```python
from build123d import *

# Parameters (mm, degrees)
F1_DEPTH      = 5
F2_ANGLE      = 30
F0_R          = 15
F4_DEPTH      = 25
F4_DEPTH_BACK = 25
F5_COUNT      = 6
F6_DEPTH      = 8.3061645655
F6_DEPTH_BACK = 8.3061645655


with BuildPart() as f1:
    # F0 (on Top) → F1 (new body, symmetric)
    with BuildSketch(Plane.XY):
        with BuildLine():
            Line((28.9777747887, -7.7645713531), (96.5925826289, -25.8819045103))
            ThreePointArc((96.5925826289, -25.8819045103), (100, 0), (96.5925826289, 25.8819045103))
            Line((96.5925826289, 25.8819045103), (28.9777747887, 7.7645713531))
            ThreePointArc((28.9777747887, 7.7645713531), (29.7433458412, 3.9157857666), (30, 0))
            ThreePointArc((30, 0), (29.7433458412, -3.9157857666), (28.9777747887, -7.7645713531))
        make_face()
        with BuildLine():
            Line((23.4384574105, -6.280315735), (28.9777747887, -7.7645713531))
            ThreePointArc((28.9777747887, -7.7645713531), (29.7433458412, -3.9157857666), (30, 0))
            ThreePointArc((30, 0), (29.7433458412, 3.9157857666), (28.9777747887, 7.7645713531))
            Line((28.9777747887, 7.7645713531), (23.4384574105, 6.280315735))
            ThreePointArc((23.4384574105, 6.280315735), (24.2652766627, 0), (23.4384574105, -6.280315735))
        make_face()
    extrude(amount=F1_DEPTH, both=True)


with BuildPart() as f1_1:
    # F2: moved
    add(f1.part.rotate(Axis((53.4821525216, 0, 0), (1, 0, 0)), F2_ANGLE))

    # F0 (on Top) → F4 (cut, two sides)
    with BuildSketch(Plane.XY) as f4_sk:
        with BuildLine():
            ThreePointArc((28.9777747887, 7.7645713531), (-30, 0), (28.9777747887, -7.7645713531))
            Line((28.9777747887, -7.7645713531), (23.4384574105, -6.280315735))
            ThreePointArc((23.4384574105, -6.280315735), (24.2652766627, 0), (23.4384574105, 6.280315735))
            Line((23.4384574105, 6.280315735), (28.9777747887, 7.7645713531))
        make_face()
        Circle(F0_R, mode=Mode.SUBTRACT)
        with BuildLine():
            Line((23.4384574105, -6.280315735), (28.9777747887, -7.7645713531))
            ThreePointArc((28.9777747887, -7.7645713531), (29.7433458412, -3.9157857666), (30, 0))
            ThreePointArc((30, 0), (29.7433458412, 3.9157857666), (28.9777747887, 7.7645713531))
            Line((28.9777747887, 7.7645713531), (23.4384574105, 6.280315735))
            ThreePointArc((23.4384574105, 6.280315735), (24.2652766627, 0), (23.4384574105, -6.280315735))
        make_face()
    extrude(amount=-F4_DEPTH, mode=Mode.SUBTRACT)
    extrude(f4_sk.sketch, amount=F4_DEPTH_BACK, mode=Mode.SUBTRACT)


with BuildPart() as f5_1:
    # F5: instance of F1
    add(f1_1.part.rotate(Axis((0, 0, 24.5690848678), (0, 0, 1)), 1 * 360 / F5_COUNT))


with BuildPart() as f5_2:
    # F5: instance of F1
    add(f1_1.part.rotate(Axis((0, 0, 24.5690848678), (0, 0, 1)), 2 * 360 / F5_COUNT))


with BuildPart() as f5_3:
    # F5: instance of F1
    add(f1_1.part.rotate(Axis((0, 0, 24.5690848678), (0, 0, 1)), 3 * 360 / F5_COUNT))


with BuildPart() as f5_4:
    # F5: instance of F1
    add(f1_1.part.rotate(Axis((0, 0, 24.5690848678), (0, 0, 1)), 4 * 360 / F5_COUNT))


with BuildPart() as f5_5:
    # F5: instance of F1
    add(f1_1.part.rotate(Axis((0, 0, 24.5690848678), (0, 0, 1)), 5 * 360 / F5_COUNT))


with BuildPart() as f1_2:
    add(f1_1.part)

    add(f5_1.part)  # F6 merges F5_1

    add(f5_2.part)  # F6 merges F5_2

    add(f5_3.part)  # F6 merges F5_3

    add(f5_4.part)  # F6 merges F5_4

    add(f5_5.part)  # F6 merges F5_5
    # F0 (on Top) → F6 (join, two sides)
    with BuildSketch(Plane.XY) as f6_sk:
        with BuildLine():
            ThreePointArc((28.9777747887, 7.7645713531), (-30, 0), (28.9777747887, -7.7645713531))
            Line((28.9777747887, -7.7645713531), (23.4384574105, -6.280315735))
            ThreePointArc((23.4384574105, -6.280315735), (24.2652766627, 0), (23.4384574105, 6.280315735))
            Line((23.4384574105, 6.280315735), (28.9777747887, 7.7645713531))
        make_face()
        Circle(F0_R, mode=Mode.SUBTRACT)
        with BuildLine():
            Line((23.4384574105, -6.280315735), (28.9777747887, -7.7645713531))
            ThreePointArc((28.9777747887, -7.7645713531), (29.7433458412, -3.9157857666), (30, 0))
            ThreePointArc((30, 0), (29.7433458412, 3.9157857666), (28.9777747887, 7.7645713531))
            Line((28.9777747887, 7.7645713531), (23.4384574105, 6.280315735))
            ThreePointArc((23.4384574105, 6.280315735), (24.2652766627, 0), (23.4384574105, -6.280315735))
        make_face()
    extrude(amount=F6_DEPTH)
    extrude(f6_sk.sketch, amount=-F6_DEPTH_BACK)


solid = f1_2.part
```
Could you check a few things on this model? Use its own coordinates, in mm. A direction names the side the tool comes from. Coordinates: 2 decimals unless noted, no trailing zeros. Write each loop counter-clockwise with the first axis right and the second up, starting at its lowest first coordinate (ties: lowest second). Pieces come first, ordered by that corner, then holes. Notation, with made-up numbers: (-7, 35.5) -> (21, 35.5) arc R34 cw to (21, 65.5) -> close; hole circle Ø8 at (82.25, 15.25). An arc over 180 degrees is marked (long way). Write item = value, one per line. Start each with the question number.
(1) I want a section at A-A (x = 0). Please give me the cut outline in (y, z).
(2) I want a section at D-D (x = 83.5). Please give me the cut outline in (y, z).
(3) Will these pins go through, and if not, where does the flat tip stop? pin 1 (3 mm diameter, centred on y = 35, z = -4, fed in from +X); pin 2 (3 mm diameter, centred on y = -57, z = 12.5, fed in from -X); pin 3 (5 mm diameter, centred on x = 13, y = 18, fed in from -Z).
(4) I need wall thicknesses on line 1 (Y direction, x = 0, z = -3.25); line 2 (X direction, y = 6.5, z = 0); line 3 (X direction, y = -37, z = -8). Which ranges of each line are inside material? Lowest first, please. Write a range as [from, to].
(5) I want a section at B-B (z = 11.5). Give the number of separate pieces and of enclosed holes in the cut face, plus the area to 3 significant figures.
(6) Which directions (+Z, -Z, +X, -X, +Y, -Y) give clear straight access to the entire face, cutting with the end or side of a thin tool? Please do faces 1 (the face through (-71.72, -2.81, -4.15)), 2 (the face through (-33.97, 63.21, 4.51)), 3 (the face through (-14, -6, 8.306)), 4 (the face through (38.3, -60.71, -4.15)).
Result set:
q1.outline = (-30, -8.31) -> (-15, -8.31) -> (-15, 8.31) -> (-30, 8.31) -> close; (15, -8.31) -> (30, -8.31) -> (30, 8.31) -> (15, 8.31) -> close
q2.outline = (-21.88, -6.86) -> (-16.88, -15.52) -> (21.88, 6.86) -> (16.88, 15.52) -> close
q3.pin_1 = 36.57
q3.pin_2 = -22.58
q3.pin_3 = -8.31
q4.line_1 = [-30, -15], [15, 30]
q4.line_2 = [-99.84, -13.52], [13.52, 99.84]
q4.line_3 = [-33.45, -25.81], [12.94, 16.91]
q5.separate_pieces = 6
q5.enclosed_holes = 0
q5.area = 1,830 mm2
q6.face_1 = -Z, -X
q6.face_2 = +Z, +Y
q6.face_3 = +Z
q6.face_4 = -Z, +X
